Autodesk Inventor part; units mm, degrees
ref_plane "YZ Plane" through (0, 0, 0) normal (1, 0, 0) x (0, 1, 0)
ref_plane "XZ Plane" through (0, 0, 0) normal (0, 1, 0) x (-1, 0, 0)
ref_plane "XY Plane" through (0, 0, 0) normal (0, 0, 1) x (1, 0, 0)
sketch "Sketch14" plane through (0, 0, 0) normal (1, 0, 0) x (0, 1, 0)
  line L0 (0, 4.9685) -> (-195, 4.9685)
  line L1 (-195, 4.9685) -> (-195, -122.0315)
  line L2 (-195, -122.0315) -> (0, -122.0315)
  line L3 (0, -122.0315) -> (0, 4.9685)
  line L4 (-6.35, -1.3815) -> (-188.65, -1.3815)
  line L5 (-188.65, -1.3815) -> (-188.65, -115.6815)
  line L6 (-188.65, -115.6815) -> (-6.35, -115.6815)
  line L7 (-6.35, -115.6815) -> (-6.35, -1.3815)
  line L8 (0, 4.9685) -> (-195, 4.9685)
  point P0 (0, 0)
extrude "Extrusion10" add sketch "Sketch14" against normal blind 254
sketch "Sketch18" plane through (-254, 0, 0) normal (-1, 0, 0) x (0, 0, 1)
  line L0 (-1.3815, -188.65) -> (-115.6815, -188.65)
  line L1 (-122.0315, 0) -> (-122.0315, -195)
  line L2 (-115.6815, -188.65) -> (-122.0315, -188.65)
  line L3 (-122.0315, -188.65) -> (-122.0315, -6.6525)
  line L4 (-122.0315, -6.6525) -> (-115.6815, -6.6525)
  line L5 (-115.6815, -6.6525) -> (-115.6815, -188.65)
  point P0 (0, 0)
extrude "Extrusion14" cut sketch "Sketch18" against normal through all
fillet "Fillet3" radius 3.175 2 edges at (-127, 0, 4.9685) (-127, -195, 4.9685)
fillet "Fillet4" radius 3.175 2 edges at (-127, 0, -122.0315) (-127, -195, -122.0315)
properties part number "WingBoxCouple"
The model under review builds one solid part; all positions refer to its coordinate system, in mm. A direction names the side the tool comes from. Round coordinates to 2 decimals unless told otherwise and drop trailing zeros. Write each loop counter-clockwise with the first axis right and the second up, starting at its lowest first coordinate (ties: lowest second). Pieces come first, ordered by that corner, then holes.
(1) Mouldability with a two-part tool opening along Z and no side actions: class faces 1 (the flat face through (-125, -96, 4.968)), 2 (the flat face through (-125, -188.65, -61)), 3 (the flat face through (-125, -6.35, -59)) as +Z half, -Z half, draft (parallel to the pull), parting line (faces both ways), or undercut.
(2) Insertion check: pin 1 (1.9 mm diameter, centred on x = -134.5, z = -120.5, fed in from -Y). The pin has a flat end and moves straight along its axis. Give the tip position at first contact, or say it passes through.
(3) Machinability: for faces 4 (the flat face through (0, -98, 3)), 5 (the flat face through (-129, -6.652, -119)), which of the approach directions +Z, -Z, +X, -X, +Y, -Y give a long, thin tool a straight path to every point of the face, cutting with its end or side? Answer none if there is none.
(4) Wall thickness on L1, parallel to Y at x = -36, z = -47.5; L2, parallel to Z at x = -19, y = -104: over which ranges is each line inside the solid? List them lowest first.
(5) We need section A-A on z = -47. Give the boundary of the cut face in (x, y).
(6) We need section C-C on y = -163. Give the boundary of the cut face in (x, z).
Findings below:
1. face 1: +Z half
1. face 2: draft
1. face 3: undercut
2. pin 1: stops at y = -194.92
3. face 4: +Z, -Z, +X, +Y, -Y
3. face 5: -Z, +X, -X
4. L1: y = -195 to -188.65, -6.35 to 0
4. L2: z = -1.38 to 4.97
5. outline: (-254, -195) - (0, -195) - (0, -188.65) - (-254, -188.65) - close; (-254, -6.35) - (0, -6.35) - (0, 0) - (-254, 0) - close
6. outline: (-254, -1.38) - (0, -1.38) - (0, 4.97) - (-254, 4.97) - close
